Could you check a few things on this model? Use its own coordinates, in mm. Face numbers are marked on the shaded views. A direction names the side the tool comes from. Round coordinates to 2 decimals unless told otherwise and drop trailing zeros. Write each loop counter-clockwise with the first axis right and the second up, starting at its lowest first coordinate (ties: lowest second). Pieces come first, ordered by that corner, then holes. Notation, with made-up numbers: M -17.75,5 L 31.25,5 A15 ccw 31.25,33 Z; hole C -14,72.25 d9. An arc over 180 degrees is marked long. One line per item, written item: value. Start each with the question number.
(1) I want a section at C-C on z = -24. Please give me the cut outline in (x, y).
(2) If I drill on L1, parallel to Y at x = 10, z = 9; L2, parallel to Z at x = 4, y = -19.5; L3, parallel to X at y = -5.5, z = -8, over which ranges is the centre line in solid material (lowest first)?
(3) I'm going to push flat-ended pins straight in: pin 1 Ø2 at (y, z) = (-27.5, 11.5) entering from +X; pin 2 Ø4 at (x, y) = (-27.5, -26) entering from +Z; pin 3 Ø5 at (y, z) = (10.24, 0) entering from -X; pin 4 Ø4 at (y, z) = (3.5, -36.5) entering from -X. Where does each tip first touch, or does it pass through?
(4) Which directions (+Z, -Z, +X, -X, +Y, -Y) give clear straight access to the entire face, cutting with the end or side of a thin tool? Please do the marked faces 5 and 6.
(5) Thinking about a two-plate mould opening in Z: for the marked faces 1, 2, 3 and 4, which applies, released by +Z, released by -Z, zero draft, split by the parting line, or undercut?
(6) I want a section at B-B on y = -12. Please give me the cut outline in (x, z), and give its area (3 significant figures).
(7) I want a section at D-D on z = 26.5. Please give me the cut outline in (x, y), and give its area (3 significant figures).
(8) I want a section at A-A on x = 0. Please give me the cut outline in (y, z), and give its area (3 significant figures).
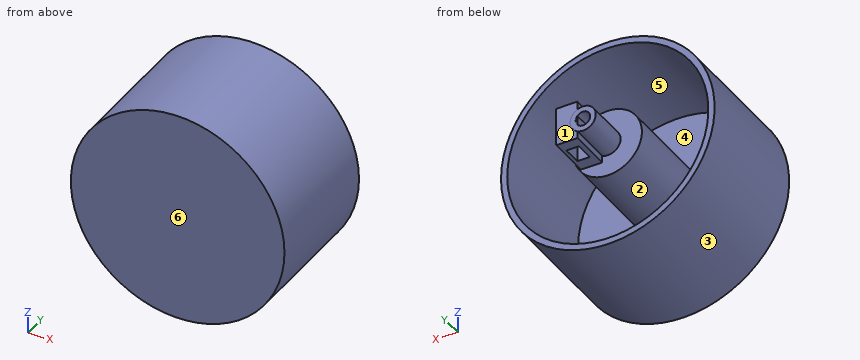
```python
from build123d import *

# Parameters (mm, degrees)
SKETCH1_R               = 6
BOSS_EXTRUDE1_DEPTH     = 20
SKETCH2_R               = 3.4
CUT_EXTRUDE1_DEPTH      = 13.55
SKETCH5_W               = 1.550685087
SKETCH5_H               = 7.184215806
BOSS_EXTRUDE2_DEPTH     = 13.55
SKETCH7_W               = 18.003976239
SKETCH7_H               = 19.909960041
BOSS_EXTRUDE3_DEPTH     = 10
SKETCH6_R               = 2
CUT_EXTRUDE2_DEPTH      = 1
CUT_EXTRUDE2_DEPTH_BACK = 13.55
CUT_EXTRUDE3_DEPTH      = 10
CUT_EXTRUDE3_DEPTH_BACK = 10
SKETCH10_R              = 50
BOSS_EXTRUDE4_DEPTH     = 60
SKETCH12_R              = 47.082764373
SKETCH12_R_2            = 15.95790089
CUT_EXTRUDE5_DEPTH      = 57


with BuildPart() as part:
    # Sketch1 → Boss-Extrude1 (new body)
    with BuildSketch(Plane(origin=(0, 0, 0), x_dir=(1, 0, 0), z_dir=(0, 1, 0))):
        Circle(SKETCH1_R)
    extrude(amount=BOSS_EXTRUDE1_DEPTH)

    # Sketch2 → Cut-Extrude1 (cut)
    with BuildSketch(Plane(origin=(0, 20, 0), x_dir=(1, 0, 0), z_dir=(0, 1, 0))):
        Circle(SKETCH2_R)
    extrude(amount=-CUT_EXTRUDE1_DEPTH, mode=Mode.SUBTRACT)

    # Sketch5 → Boss-Extrude2 (add)
    with BuildSketch(Plane(origin=(0, 18.26, 0), x_dir=(1, 0, 0), z_dir=(0, 1, 0))):
        with Locations((3.375342544, 0.020519704)):
            Rectangle(SKETCH5_W, SKETCH5_H)
    extrude(amount=-BOSS_EXTRUDE2_DEPTH)

    # Sketch7 → Boss-Extrude3 (add)
    with BuildSketch(Plane.ZY.offset(-2.6)):
        with Locations((0.33027221, 9.954980021)):
            Rectangle(SKETCH7_W, SKETCH7_H)
    extrude(amount=-BOSS_EXTRUDE3_DEPTH)

    # Sketch6 → Cut-Extrude2 (cut, two sides)
    with BuildSketch(Plane.ZY.offset(-2.6)) as cut_extrude2_sk:
        with Locations((0, 10.236925537)):
            Circle(SKETCH6_R)
    extrude(amount=CUT_EXTRUDE2_DEPTH, mode=Mode.SUBTRACT)
    extrude(cut_extrude2_sk.sketch, amount=-CUT_EXTRUDE2_DEPTH_BACK, mode=Mode.SUBTRACT)

    # Sketch9 → Cut-Extrude3 (cut, two sides)
    with BuildSketch(Plane.XY) as cut_extrude3_sk:
        Polygon((10.876516382, 10.236925537), (10.876516382, 5.861925537), (4.943430227, 5.861925537), (4.943430227, 10.236925537), (4.943430227, 14.614332445), (10.876516382, 14.614332445), align=None)
    extrude(amount=CUT_EXTRUDE3_DEPTH, mode=Mode.SUBTRACT)
    extrude(cut_extrude3_sk.sketch, amount=-CUT_EXTRUDE3_DEPTH_BACK, mode=Mode.SUBTRACT)

    # Sketch10 → Boss-Extrude4 (add)
    with BuildSketch(Plane.XZ):
        Circle(SKETCH10_R)
    extrude(amount=BOSS_EXTRUDE4_DEPTH)

    # Sketch12 → Cut-Extrude5 (cut)
    with BuildSketch(Plane(origin=(0, 0, 0), x_dir=(1, 0, 0), z_dir=(0, 1, 0))):
        Circle(SKETCH12_R)
        Circle(SKETCH12_R_2, mode=Mode.SUBTRACT)
    extrude(amount=-CUT_EXTRUDE5_DEPTH, mode=Mode.SUBTRACT)


solid = part.part
```
Found:
1. outline: M -43.86,-60 L 43.86,-60 L 43.86,0 L 40.51,0 L 40.51,-57 L -40.51,-57 L -40.51,0 L -43.86,0 Z
2. L1: y = -60 to 5.86, 14.61 to 19.91
2. L2: z = -49.84 to -46.91, -15.45 to 15.45, 46.91 to 49.84
2. L3: x = -49.36 to -46.4, -13.81 to 13.81, 46.4 to 49.36
3. pin 1: stops at x = 48.89
3. pin 2: stops at z = 43.01
3. pin 3: stops at x = -6
3. pin 4: passes through
4. face 5: +Y
4. face 6: +Z, -Z, +X, -X, -Y
5. face 1: zero draft
5. face 2: undercut
5. face 3: split by the parting line
5. face 4: undercut
6. outline: C 0,0 d100; C 0,0 d31.92; hole C 0,0 d94.17
6. area: 1,690 mm²
7. outline: M -42.4,-60 L 42.4,-60 L 42.4,0 L 38.92,0 L 38.92,-57 L -38.92,-57 L -38.92,0 L -42.4,0 Z
7. area: 651 mm²
8. outline: M -60,-50 L 0,-50 L 0,-47.08 L -57,-47.08 L -57,-15.96 L 0,-15.96 L 0,-6 L 20,-6 L 20,-3.4 L 6.45,-3.4 L 6.45,3.4 L 20,3.4 L 20,6 L 0,6 L 0,15.96 L -57,15.96 L -57,47.08 L 0,47.08 L 0,50 L -60,50 Z
8. area: 2,600 mm²
